```python
from build123d import *

# Parameters (mm, degrees)
SKETCH1_W                 = 199
SKETCH1_H                 = 41
BOSS_EXTRUDE1_DEPTH       = 52.5
SKETCH10_W                = 25.4
SKETCH10_H                = 89.125
BOSS_EXTRUDE6_DEPTH       = 17
M4X0_7_TAPPED_HOLE1_D     = 3.3
M4X0_7_TAPPED_HOLE1_DEPTH = 9.906
M4X0_7_TAPPED_HOLE1_TIP   = 0.991420021


with BuildPart() as part:
    # Sketch1 → Boss-Extrude1 (new, symmetric)
    with BuildSketch(Plane(origin=(0, 0, 0), x_dir=(1, 0, 0), z_dir=(0, 1, 0))):
        Rectangle(SKETCH1_W, SKETCH1_H)
    extrude(amount=BOSS_EXTRUDE1_DEPTH, both=True)

    # Sketch10 → Boss-Extrude6 (add)
    with BuildSketch(Plane(origin=(99.5, 0, 0), x_dir=(0, 0, -1), z_dir=(1, 0, 0))):
        with Locations((-1.45, 4.7625)):
            Rectangle(SKETCH10_W, SKETCH10_H)
    extrude(amount=BOSS_EXTRUDE6_DEPTH)

    # M4x0.7 Tapped Hole1
    with Locations(Plane.XY.offset(20.5)):
        with Locations((-57, 37.5), (63, -37.5), (-57, -37.5), (63, 37.5)):
            Hole(M4X0_7_TAPPED_HOLE1_D / 2, depth=M4X0_7_TAPPED_HOLE1_DEPTH)
            with Locations((0, 0, -(M4X0_7_TAPPED_HOLE1_DEPTH + M4X0_7_TAPPED_HOLE1_TIP / 2))):  # 118° drill point
                Cone(0, M4X0_7_TAPPED_HOLE1_D / 2, M4X0_7_TAPPED_HOLE1_TIP, mode=Mode.SUBTRACT)


solid = part.part
```
Part model, mm, in its own coordinate system. A direction names the side the tool comes from. Give positions to 0.01 mm unless a question says otherwise; leave off trailing zeros. Write each loop counter-clockwise with the first axis right and the second up, starting at its lowest first coordinate (ties: lowest second). Pieces come first, ordered by that corner, then holes. Notation, with made-up numbers: (32, 63.25) -> (70, 63.25) arc R23 cw to (70, 79.25) -> close; hole circle Ø6 at (-30, 56). An arc over 180 degrees is marked (long way). Put each result on its own line as item: value. Start each with the question number.
Item 1: Pull direction X, two halves, no side cores. Call faces 1 (the face through (116.5, 5, 2)), 2 (the face through (-99.5, 1, 0)), 3 (the face through (108, 49.325, 2)): pulls with the +X half, pulls with the -X half, needs draft (parallel to the pull), parting line crosses it, or undercut.
Item 2: Wall check: L1, parallel to X at y = -37.5, z = 16.25; L2, parallel to Y at x = 63, z = 14; L3, parallel to X at y = 37, z = 13. Give the ranges that are in metal, low to high. Write a range as [from, to].
Item 3: Cut at A-A (y = 15.5). List the corners of the cut face in (x, z), then the cut area to 3 significant figures.
Item 4: Pin check, flat tips, straight feed: pin 1 Ø18.5 at (x, y) = (104.5, 6) entering from +Z; pin 2 Ø3 at (x, y) = (-57, -37.5) entering from +Z; pin 3 Ø13.5 at (x, z) = (106.5, 3) entering from +Y (3 decimals); pin 4 Ø8.5 at (x, y) = (106, 2.5) entering from -Z. Stop position of each tip, or through.
Item 5: Which spindle directions (+Z, -Z, +X, -X, +Y, -Y) get a long thin tool onto all of the face, cutting with end or side? Do faces 4 (the face through (108, -39.8, 2)), 5 (the face through (-1, 1, -20.5)), 6 (the face through (108, 4, 14.15)), 7 (the face through (108, 4, -11.25)), 8 (the face through (-1, -52.5, 0)). Say none if no direction does.
Answer list:
1. face 1: pulls with the +X half
1. face 2: pulls with the -X half
1. face 3: needs draft
2. L1: x = [-99.5, -58.65], [-55.35, 61.35], [64.65, 99.5]
2. L2: y = [-52.5, -39.15], [-35.85, 35.85], [39.15, 52.5]
2. L3: x = [-99.5, -58.57], [-55.43, 61.43], [64.57, 116.5]
3. outline: (-99.5, -20.5) -> (99.5, -20.5) -> (99.5, -11.25) -> (116.5, -11.25) -> (116.5, 14.15) -> (99.5, 14.15) -> (99.5, 20.5) -> (-99.5, 20.5) -> close
3. area: 8,590 mm2
4. pin 1: stops at z = 20.5
4. pin 2: stops at z = 10.5
4. pin 3: stops at y = 49.325
4. pin 4: stops at z = -11.25
5. face 4: +Z, -Z, +X, -Y
5. face 5: -Z, +X, -X, +Y, -Y
5. face 6: +Z, +X, +Y, -Y
5. face 7: -Z, +X, +Y, -Y
5. face 8: +Z, -Z, +X, -X, -Y
